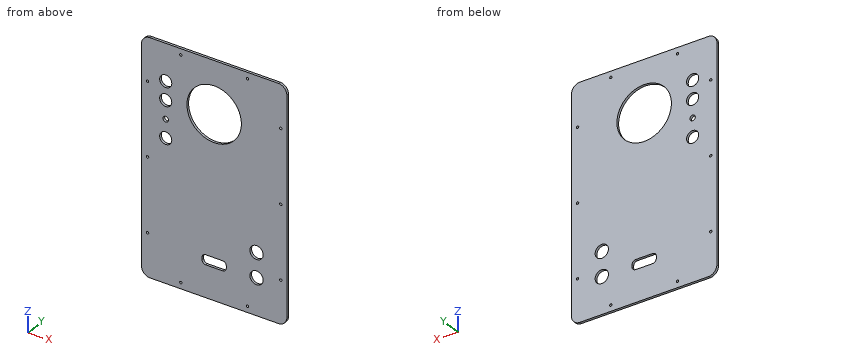
```python
from build123d import *

# Parameters (mm, degrees)
F0_R     = 5.5
F0_R_2   = 5
F0_R_3   = 2.25
F0_R_4   = 22.5
F1_DEPTH = 2
F2_D     = 2


with BuildPart() as f1:
    # F0 (on Front) → F1 (new body)
    with BuildSketch(Plane.XZ):
        with BuildLine():
            ThreePointArc((60, 88), (57.949747, 92.949747), (53, 95))
            Line((53, 95), (-53, 95))
            ThreePointArc((-53, 95), (-57.949747, 92.949747), (-60, 88))
            Line((-60, 88), (-60, -88))
            ThreePointArc((-60, -88), (-57.949747, -92.949747), (-53, -95))
            Line((-53, -95), (53, -95))
            ThreePointArc((53, -95), (57.949747, -92.949747), (60, -88))
            Line((60, -88), (60, 88))
        make_face()
        with BuildLine():
            ThreePointArc((10, -66), (9.12132, -68.12132), (7, -69))
            Line((7, -69), (-7, -69))
            ThreePointArc((-7, -69), (-9.12132, -68.12132), (-10, -66))
            Line((-10, -66), (-10, -64))
            ThreePointArc((-10, -64), (-9.12132, -61.87868), (-7, -61))
            Line((-7, -61), (7, -61))
            ThreePointArc((7, -61), (9.12132, -61.87868), (10, -64))
            Line((10, -64), (10, -66))
        make_face(mode=Mode.SUBTRACT)
        with Locations((35, -65)):
            Circle(F0_R, mode=Mode.SUBTRACT)
        with Locations((35, -45)):
            Circle(F0_R, mode=Mode.SUBTRACT)
        with Locations((-40, 20)):
            Circle(F0_R_2, mode=Mode.SUBTRACT)
        with Locations((-40, 35)):
            Circle(F0_R_3, mode=Mode.SUBTRACT)
        with Locations((-40, 50)):
            Circle(F0_R_2, mode=Mode.SUBTRACT)
        with Locations((-40, 65)):
            Circle(F0_R_2, mode=Mode.SUBTRACT)
        with Locations((0, 52.5)):
            Circle(F0_R_4, mode=Mode.SUBTRACT)
    extrude(amount=F1_DEPTH)

    # F2 (through all)
    with Locations(Plane(origin=(0, 0, 0), x_dir=(1, 0, 0), z_dir=(0, 1, 0))):
        with Locations((-27.5, 90), (-55, 60), (-55, 0), (-55, -60), (-27.5, -90), (27.5, -90), (55, -60), (55, 0), (55, 60), (27.5, 90)):
            Hole(F2_D / 2)


solid = f1.part
```
Design review of the part built by this model. Coordinates are the model's own, in mm. Coordinates: 2 decimals unless noted, no trailing zeros. Order: outer loops, then holes, each group sorted by start corner. A loop starts at its lowest first (then second) coordinate and runs counter-clockwise, first axis right, second up. Notation, with made-up numbers: (23, 47.25) - (39, 47.25) arc R27 cw to (39, 84.25) - close; hole circle Ø10 at (27, -4). An arc over 180 degrees is marked (long way). Answer in a Markdown table with one row per item.
(1) Consider section C-C on y = -0.9. Give the number of separate pieces and of enclosed holes in the cut face, plus the area to 3 significant figures.
Checked values:
| item | result |
|---|---|
| separate pieces | 1 |
| enclosed holes | 18 |
| area | 20,500 mm^2 |
(2) Consider section A-A on x = 0. State the section outline as (y, z) points.
Checked values:
| item | result |
|---|---|
| outline | (-2, -95) - (0, -95) - (0, -69) - (-2, -69) - close; (-2, -61) - (0, -61) - (0, 30) - (-2, 30) - close; (-2, 75) - (0, 75) - (0, 95) - (-2, 95) - close |
(3) Wall thickness on line 1 along Z through (x, y) = (-40, -0.65); line 2 along Z through (x, y) = (35, -0.9); line 3 along X through (y, z) = (-0.65, 47): over which ranges is each line inside the solid? List them lowest first. Write a range as from..to.
Checked values:
| item | result |
|---|---|
| line 1 | -95..15, 25..32.75, 37.25..45, 55..60, 70..95 |
| line 2 | -95..-70.5, -59.5..-50.5, -39.5..95 |
| line 3 | -60..-44, -36..-21.82, 21.82..60 |
(4) Consider section B-B on z = 20. State the section outline as (x, y) points, plus the area to 3 significant figures.
Checked values:
| item | result |
|---|---|
| outline | (-60, -2) - (-45, -2) - (-45, 0) - (-60, 0) - close; (-35, -2) - (60, -2) - (60, 0) - (-35, 0) - close |
| area | 220 mm^2 |
(5) Consider section D-D on x = 34. State the section outline as (y, z) points, plus the area to 3 significant figures.
Checked values:
| item | result |
|---|---|
| outline | (-2, -95) - (0, -95) - (0, -70.41) - (-2, -70.41) - close; (-2, -59.59) - (0, -59.59) - (0, -50.41) - (-2, -50.41) - close; (-2, -39.59) - (0, -39.59) - (0, 95) - (-2, 95) - close |
| area | 337 mm^2 |
